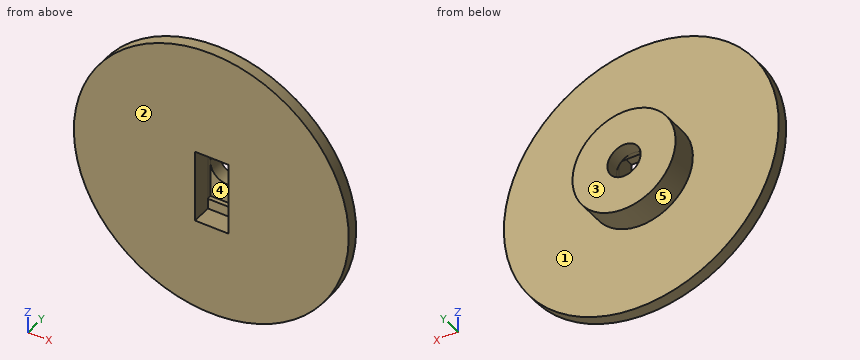
```python
from build123d import *

# Parameters (mm, degrees)
SKETCH1_R           = 60
BOSS_EXTRUDE1_DEPTH = 5
SKETCH2_R           = 22.5
BOSS_EXTRUDE3_DEPTH = 11.7
SKETCH6_R           = 7.25
CUT_EXTRUDE4_DEPTH  = 6
SKETCH7_W           = 14.5
SKETCH7_H           = 22.8
CUT_EXTRUDE5_DEPTH  = 2
SKETCH9_W           = 14.5
SKETCH9_H           = 31.8
CUT_EXTRUDE6_DEPTH  = 25


with BuildPart() as part:
    # Sketch1 → Boss-Extrude1 (new body)
    with BuildSketch(Plane(origin=(0, 0, 0), x_dir=(1, 0, 0), z_dir=(0, 1, 0))):
        with Locations(Location((0, 0, 0), (0, 0, 270))):
            Circle(SKETCH1_R)
    extrude(amount=BOSS_EXTRUDE1_DEPTH)

    # Sketch2 → Boss-Extrude3 (add)
    with BuildSketch(Plane(origin=(0, 5, 0), x_dir=(1, 0, 0), z_dir=(0, 1, 0))):
        with Locations(Location((0, 0, 0), (0, 0, 270))):
            Circle(SKETCH2_R)
    extrude(amount=BOSS_EXTRUDE3_DEPTH)

    # Sketch6 → Cut-Extrude4 (cut)
    with BuildSketch(Plane(origin=(0, 16.7, 0), x_dir=(1, 0, 0), z_dir=(0, 1, 0))):
        with Locations(Location((0, 0, 0), (0, 0, 270))):
            Circle(SKETCH6_R)
    extrude(amount=-CUT_EXTRUDE4_DEPTH, mode=Mode.SUBTRACT)

    # Sketch7 → Cut-Extrude5 (cut)
    with BuildSketch(Plane(origin=(0, 10.7, 0), x_dir=(1, 0, 0), z_dir=(0, 1, 0))):
        with Locations((0, 4.15)):
            Rectangle(SKETCH7_W, SKETCH7_H)
    extrude(amount=-CUT_EXTRUDE5_DEPTH, mode=Mode.SUBTRACT)

    # Sketch9 → Cut-Extrude6 (cut)
    with BuildSketch(Plane(origin=(0, 8.7, 0), x_dir=(1, 0, 0), z_dir=(0, 1, 0))):
        with Locations((0.153398413, 4.15)):
            Rectangle(SKETCH9_W, SKETCH9_H)
    extrude(amount=-CUT_EXTRUDE6_DEPTH, mode=Mode.SUBTRACT)


solid = part.part
```
The listing builds one solid part. Answer for the finished solid, in the listing's coordinates (mm). Face numbers are marked on the shaded views. A direction names the side the tool comes from. Round coordinates to 2 decimals unless told otherwise and drop trailing zeros. Loops run counter-clockwise (first coordinate to the right, second up) from the corner with the lowest first, then second, coordinate; pieces in that order, holes last.
Q1. Given pin 1 Ø6 at (x, y) = (12, 12.5) entering from +Z; pin 2 Ø1 at (x, y) = (-2, 9.5) entering from -Z; pin 3 Ø6 at (y, z) = (12.5, 0) entering from +X, each flat-ended and moving along its own axis, determine where each tip first touches the part or whether it passes through.
Q2. Section C-C, the plane z = 37 is taken. Determine the outline of the cut face in (x, y), then the cut area to 3 significant figures.
Q3. Section B-B, the plane x = -11 is taken. Determine the outline of the cut face in (y, z), then the cut area to 3 significant figures.
Q4. Find the intervals of material crossed by line 1 (X direction, y = 13.35, z = 0); line 2 (Y direction, x = -42.5, z = -3.5); line 3 (Z direction, x = 6, y = 6), in increasing order.
Q5. Section D-D, the plane x = 16 is taken. Determine the outline of the cut face in (y, z).
Q6. For a pull along X with two mould halves and no side action, classify the marked faces 3, 4 and 5 as released by +X, released by -X, zero draft, split by the parting line, or undercut.
Q7. Which of the six approach directions +Z, -Z, +X, -X, +Y, -Y give full straight-line access (tool end or side, diameter ignored) to the marked faces 1 and 2?
Q8. Section A-A, the plane y = 14.25 is taken. Determine the outline of the cut face in (x, z).
Completed:
1. pin 1: stops at z = 20.62
1. pin 2: stops at z = -22.45
1. pin 3: stops at x = 22.5
2. outline: (-47.23, 0) - (47.23, 0) - (47.23, 5) - (-47.23, 5) - close
2. area: 472 mm2
3. outline: (0, -58.98) - (5, -58.98) - (5, -19.63) - (16.7, -19.63) - (16.7, 19.63) - (5, 19.63) - (5, 58.98) - (0, 58.98) - close
3. area: 1,050 mm2
4. line 1: x = -22.5 to -7.25, 7.25 to 22.5
4. line 2: y = 0 to 5
4. line 3: z = -21.69 to -20.05, 11.75 to 21.69
5. outline: (0, -57.83) - (5, -57.83) - (5, -15.82) - (16.7, -15.82) - (16.7, 15.82) - (5, 15.82) - (5, 57.83) - (0, 57.83) - close
6. face 3: zero draft
6. face 4: undercut
6. face 5: split by the parting line
7. face 1: +Y
7. face 2: +Z, -Z, +X, -X, -Y
8. outline: circle Ø45 at (0, 0); hole circle Ø14.5 at (0, 0)
